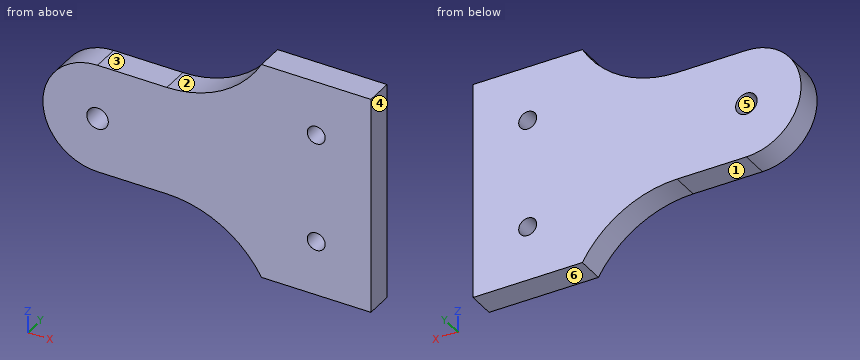
from build123d import *

# Parameters (mm, degrees)
BOSS_EXTRUDE1_DEPTH = 6.35
FILLET1_R           = 25.4
SKETCH2_R           = 2.5
CUT_EXTRUDE1_DEPTH  = 6.35
SKETCH3_R           = 2.0828
CUT_EXTRUDE2_DEPTH  = 6.35


with BuildPart() as part:
    # Sketch1 → Boss-Extrude1 (new body)
    with BuildSketch(Plane(origin=(0, 0, 0), x_dir=(1, 0, 0), z_dir=(0, 1, 0))):
        with BuildLine():
            Line((0, 12.7), (38.1, 12.7))
            Line((38.1, 12.7), (38.1, 25.4))
            Line((38.1, 25.4), (63.5, 25.4))
            Line((63.5, 25.4), (63.5, -25.4))
            Line((63.5, -25.4), (38.1, -25.4))
            Line((38.1, -25.4), (38.1, -12.7))
            Line((38.1, -12.7), (0, -12.7))
            ThreePointArc((0, -12.7), (-12.7, 0), (0, 12.7))
        make_face()
    extrude(amount=BOSS_EXTRUDE1_DEPTH)

    # Fillet1
    # the kernel refuses this fillet: 25.4 mm, written as the material it adds along each edge
    with BuildSketch(Plane(origin=(38.1, 0, 12.7), x_dir=(0, 0, 1), z_dir=(0, 1, 0))) as fillet1_piece_1:
        with BuildLine():
            CenterArc((25.4, -21.997045256), FILLET1_R, 120, 60)
            Line((0, -21.997045256), (-0.508, -21.997045256))
            Line((-0.508, -21.997045256), (-0.508, 0))
            Line((-0.508, 0), (0, 0.508))
            ThreePointArc((0, 0.508), (6.35, 0.508), (12.446, 0.439940905))
            Line((12.446, 0.439940905), (12.7, 0))
        make_face()
    extrude(amount=6.35)
    with BuildSketch(Plane(origin=(38.1, 0, -12.7), x_dir=(-1, 0, 0), z_dir=(0, 1, 0))) as fillet1_piece_2:
        with BuildLine():
            CenterArc((21.997045256, -25.4), FILLET1_R, 90, 60)
            Line((0, -12.7), (-0.439940905, -12.446))
            ThreePointArc((-0.439940905, -12.446), (-0.508, -6.35), (-0.508, 0))
            Line((-0.508, 0), (0, 0.508))
            Line((0, 0.508), (21.997045256, 0.508))
            Line((21.997045256, 0.508), (21.997045256, 0))
        make_face()
    extrude(amount=6.35)

    # Sketch2 → Cut-Extrude1 (cut)
    with BuildSketch(Plane(origin=(0, 6.35, 0), x_dir=(1, 0, 0), z_dir=(0, 1, 0))):
        with Locations(Location((0, 0, 0), (0, 0, 270))):
            Circle(SKETCH2_R)
    extrude(amount=-CUT_EXTRUDE1_DEPTH, mode=Mode.SUBTRACT)

    # Sketch3 → Cut-Extrude2 (cut)
    with BuildSketch(Plane(origin=(0, 6.35, 0), x_dir=(1, 0, 0), z_dir=(0, 1, 0))):
        with Locations(Location((50.8, 12.7, 0), (0, 0, 270))):
            Circle(SKETCH3_R)
        with Locations(Location((50.8, -12.7, 0), (0, 0, 270))):
            Circle(SKETCH3_R)
    extrude(amount=-CUT_EXTRUDE2_DEPTH, mode=Mode.SUBTRACT)


solid = part.part
Design review of the part built by this model. Coordinates are the model's own, in mm. Face numbers are marked on the shaded views. A direction names the side the tool comes from. Round coordinates to 2 decimals unless told otherwise and drop trailing zeros. Order: outer loops, then holes, each group sorted by start corner. A loop starts at its lowest first (then second) coordinate and runs counter-clockwise, first axis right, second up.
1) Machinability: for the marked faces 1 and 2, which of the approach directions +Z, -Z, +X, -X, +Y, -Y give a long, thin tool a straight path to every point of the face, cutting with its end or side? Answer none if there is none.
The answers:
face 1: -Z, -X, +Y, -Y
face 2: +Z, -X, +Y, -Y
2) Consider section C-C (z = 13.5). State the section outline as (x, y) points.
The answers:
outline: (22.43, 0) - (48.88, 0) - (48.88, 6.35) - (22.43, 6.35) - close; (52.72, 0) - (63.5, 0) - (63.5, 6.35) - (52.72, 6.35) - close
3) For L1, parallel to X at y = 6, z = -11; L2, parallel to X at y = 4.75, z = -6.5; L3, parallel to X at y = 1.25, z = 9.5, list the stretches that pass through material, from the lowest coordinate up.
The answers:
L1: x = -6.35 to 49.6, 52 to 63.5
L2: x = -10.91 to 63.5
L3: x = -8.43 to 63.5
4) Consider section D-D (z = -6.5). State the section outline as (x, y) points, plus the area to 3 significant figures.
The answers:
outline: (-10.91, 0) - (63.5, 0) - (63.5, 6.35) - (-10.91, 6.35) - close
area: 473 mm2
5) Draft analysis for pull direction Z (two halves, no side actions). For the marked faces 3, 4, 5 and 6, state which applies: released by +Z, released by -Z, zero draft, split by the parting line, or undercut.
The answers:
face 3: released by +Z
face 4: zero draft
face 5: undercut
face 6: released by -Z
6) Consider section B-B (y = 3). State the section outline as (x, z) points.
The answers:
outline: (0, -12.7) - (16.1, -12.7) arc R25.4 cw to (38.1, -25.4) - (63.5, -25.4) - (63.5, 25.4) - (38.1, 25.4) arc R25.4 cw to (16.1, 12.7) - (0, 12.7) arc R12.7 ccw to start; hole circle Ø5 at (0, 0); hole circle Ø4.17 at (50.8, -12.7); hole circle Ø4.17 at (50.8, 12.7)
7) Consider section A-A (x = 50.8). State the section outline as (y, z) points, plus the area to 3 significant figures.
The answers:
outline: (0, -25.4) - (6.35, -25.4) - (6.35, -14.78) - (0, -14.78) - close; (0, -10.62) - (6.35, -10.62) - (6.35, 10.62) - (0, 10.62) - close; (0, 14.78) - (6.35, 14.78) - (6.35, 25.4) - (0, 25.4) - close
area: 270 mm2
8) Clearance check with flat-ended pins moving along their axes: pin 1 Ø1.9 at (x, y) = (12, 4.5) entering from +Z; pin 2 Ø1.9 at (x, y) = (7, 4.5) entering from -Z; pin 3 Ø3 at (x, y) = (28.5, 3.5) entering from -Z. State where each tip first meets the part, or that it passes through.
The answers:
pin 1: stops at z = 12.7
pin 2: stops at z = -12.7
pin 3: stops at z = -16.84
